from build123d import *

# Parameters (mm, degrees)
SKETCH1_R           = 1.2
SKETCH1_R_2         = 1
BOSS_EXTRUDE1_DEPTH = 2.4
CUT_EXTRUDE1_DEPTH  = 24.69949444


with BuildPart() as part:
    # Sketch1 → Boss-Extrude1 (new body)
    with BuildSketch(Plane(origin=(0, 0, 0), x_dir=(1, 0, 0), z_dir=(0, 1, 0))):
        with BuildLine():
            Line((-12.181045185, 8), (22.178954815, 8))
            Line((22.178954815, 8), (12.181045185, -8))
            Line((12.181045185, -8), (-12.181045185, -8))
            ThreePointArc((-12.181045185, -8), (-20.181045185, 0), (-12.181045185, 8))
        make_face()
        with Locations(Location((-12.181045185, 4.5, 0), (0, 0, 270))):
            Circle(SKETCH1_R, mode=Mode.SUBTRACT)
        with Locations(Location((-7.681045185, 0, 0), (0, 0, 270))):
            Circle(SKETCH1_R, mode=Mode.SUBTRACT)
        with Locations(Location((-12.181045185, -4.5, 0), (0, 0, 270))):
            Circle(SKETCH1_R, mode=Mode.SUBTRACT)
        with Locations(Location((-16.681045185, 0, 0), (0, 0, 270))):
            Circle(SKETCH1_R, mode=Mode.SUBTRACT)
        with Locations(Location((18.029644978, 5.7, 0), (0, 0, 270))):
            Circle(SKETCH1_R, mode=Mode.SUBTRACT)
        with Locations(Location((13.2603716, -1.932432865, 0), (0, 0, 270))):
            Circle(SKETCH1_R, mode=Mode.SUBTRACT)
        with Locations(Location((15.645008289, 1.883783567, 0), (0, 0, 270))):
            Circle(SKETCH1_R, mode=Mode.SUBTRACT)
        with Locations(Location((-12.181045185, 0, 0), (0, 0, 270))):
            Circle(SKETCH1_R_2, mode=Mode.SUBTRACT)
    extrude(amount=BOSS_EXTRUDE1_DEPTH)

    # Sketch2 → Cut-Extrude1 (cut, through all)
    with BuildSketch(Plane(origin=(0, 2.4, 0), x_dir=(1, 0, 0), z_dir=(0, 1, 0))):
        with BuildLine():
            Line((14.535282418, -4.232432865), (-5.392340445, -4.232432865))
            ThreePointArc((-5.392340445, -4.232432865), (-8.299000809, -6.994979018), (-12.181045185, -8))
            Line((-12.181045185, -8), (12.181045185, -8))
            Line((12.181045185, -8), (14.535282418, -4.232432865))
        make_face()
    extrude(amount=-CUT_EXTRUDE1_DEPTH, mode=Mode.SUBTRACT)


solid = part.part
Work out the finished part from the listing and answer in its coordinate system (mm). A direction names the side the tool comes from. Coordinates: 2 decimals unless noted, no trailing zeros. Write each loop counter-clockwise with the first axis right and the second up, starting at its lowest first coordinate (ties: lowest second). Pieces come first, ordered by that corner, then holes. Notation, with made-up numbers: (31, 71.25) - (61, 71.25) arc R21 cw to (61, 89.25) - close; hole circle Ø8 at (78.25, 15.25). An arc over 180 degrees is marked (long way). One line per question, with ' | ' between items.
1) Find section D-D, the plane y = 0.7. Give the number of separate pieces and of enclosed holes in the cut face, and give its area (3 significant figures).
Checks:
separate pieces: 1 | enclosed holes: 8 | area: 457 mm2
2) For faces 1 (the face through (-15.49, 1.18, -0.16)), 2 (the face through (5, 1, 4.232)), determine the directions among +Z, -Z, +X, -X, +Y, -Y from which every point of the face is accessible in a straight line to the end or side of a thin tool.
Checks:
face 1: +Y, -Y | face 2: +Z, +X, +Y, -Y
3) Find section B-B, the plane x = 17.5. Determine the outline of the cut face in (y, z), and give its area (3 significant figures).
Checks:
outline: (0, -8) - (2.4, -8) - (2.4, -6.78) - (0, -6.78) - close; (0, -4.62) - (2.4, -4.62) - (2.4, -0.51) - (0, -0.51) - close | area: 12.8 mm2
4) Flat-ended cylindrical pins translate along their axes: P1, Ø3, axis at x = -12.18, z = 4.5, coming from the +Y side; P2, Ø2, axis at x = 18.03, z = -5.7, coming from the -Y side. Find the tip coordinate at first contact, or state that the pin passes through.
Checks:
P1: y = 2.4 | P2: through
5) Find section C-C, the plane z = 4.75. Determine the outline of the cut face in (x, y).
Checks:
outline: (-18.62, 0) - (-13.35, 0) - (-13.35, 2.4) - (-18.62, 2.4) - close; (-11.01, 0) - (-5.74, 0) - (-5.74, 2.4) - (-11.01, 2.4) - close
6) Find section A-A, the plane z = 0. Determine the outline of the cut face in (x, y), and give its area (3 significant figures).
Checks:
outline: (-20.18, 0) - (-17.88, 0) - (-17.88, 2.4) - (-20.18, 2.4) - close; (-15.48, 0) - (-13.18, 0) - (-13.18, 2.4) - (-15.48, 2.4) - close; (-11.18, 0) - (-8.88, 0) - (-8.88, 2.4) - (-11.18, 2.4) - close; (-6.48, 0) - (17.18, 0) - (17.18, 2.4) - (-6.48, 2.4) - close | area: 73.3 mm2
7) The mould has two halves that part along Z. Classify faces 3 (the face through (-8.853, 1.183, -0.26)), 4 (the face through (1, 2.4, -2)), 5 (the face through (18.41, 1.18, -1.97)): +Z half, -Z half, draft (parallel to the pull), parting line (faces both ways), or undercut.
Checks:
face 3: undercut | face 4: draft | face 5: +Z half
8) Consider probe 1 along X at (y, z) = (1.3, -0.5); probe 2 along Z at (x, y) = (-12, 1.75); probe 3 along Z at (x, y) = (5, 1.65). Determine where each line is inside the solid, lowest interval first. Write a range as [from, to].
Checks:
probe 1: [-20.17, -17.77], [-15.59, -13.05], [-11.32, -8.77], [-6.59, 17.49] | probe 2: [-8, -5.69], [-3.31, -0.98], [0.98, 3.31], [5.69, 8] | probe 3: [-8, 4.23]
